Geometry check sheet. Reference: the model listing, model coordinates, mm. Face numbers are marked on the shaded views. A direction names the side the tool comes from. Give positions to 0.01 mm unless a question says otherwise; leave off trailing zeros. Order: outer loops, then holes, each group sorted by start corner. A loop starts at its lowest first (then second) coordinate and runs counter-clockwise, first axis right, second up. Notation, with made-up numbers: M 3.5,53 L 56.5,53 A22 cw 56.5,81 Z; hole C 60,33.25 d1. An arc over 180 degrees is marked long. Answer as CSV lines item,"result". Start each with the question number.
Q1. Section check B-B, the plane x = -50. Record the boundary of the cut face in (y, z).
Q2. Section check C-C, the plane x = -86. Record the boundary of the cut face in (y, z).
Q3. Go/stop test with flat-tipped pins: pin 1 (6 mm diameter, centred on x = -65, y = 16.5, fed in from +Z); pin 2 (5 mm diameter, centred on x = -80, y = 9.95, fed in from -Z); pin 3 (1.4 mm diameter, centred on y = 21.5, z = 1, fed in from +X); pin 4 (1.5 mm diameter, centred on x = -33.5, z = 1.5, fed in from -Y). Record where each tip stops, or that it passes through.
Q4. Section check A-A, the plane y = 16. Record the boundary of the cut face in (x, z).
Q5. Thickness scan on line 1 (Y direction, x = -70, z = 0.85); line 2 (Z direction, x = -87, y = 2.5); line 3 (X direction, y = 1.75, z = 0.95). Record the ranges inside material, lowest first.
Q6. Set-up check for the marked faces 1 and 2: record each of +Z, -Z, +X, -X, +Y, -Y from which the full face is reachable in a straight line by a thin tool's end or side.
```python
from build123d import *

# Parameters (mm, degrees)
F0_W      = 96
F0_H      = 20
F1_DEPTH  = 2.4
F4_DEPTH  = 20
F5_R      = 0.75
F6_DEPTH  = 20.001
F7_R      = 1.5
F8_DEPTH  = 2.401
F10_DEPTH = 2.4
F11_DEPTH = 2.401


with BuildPart() as f1:
    # F0 (on Top) → F1 (new body)
    with BuildSketch(Plane.XY):
        with Locations((-48, 10)):
            Rectangle(F0_W, F0_H)
    extrude(amount=F1_DEPTH)

    # F3 (on face) → F4 (join)
    with BuildSketch(Plane.XZ):
        with BuildLine():
            Line((-4.53507, 2.4), (0, 2.4))
            Line((0, 2.4), (0, 4.9))
            Line((0, 4.9), (-2.557698, 4.9))
            ThreePointArc((-2.557698, 4.9), (-3.861539, 4.416575), (-4.53507, 3.2))
            ThreePointArc((-4.53507, 3.2), (-4.769385, 2.634315), (-5.33507, 2.4))
            Line((-5.33507, 2.4), (-4.53507, 2.4))
        make_face()
    extrude(amount=-F4_DEPTH)

    # F5 (on face) → F6 (cut, through all)
    with BuildSketch(Plane.XZ):
        with Locations((-2.673816, 2.433896)):
            Circle(F5_R)
    extrude(amount=-F6_DEPTH, mode=Mode.SUBTRACT)

    # F7 (on face) → F8 (cut, through all)
    with BuildSketch(Plane.XY.offset(2.4)):
        with BuildLine():
            ThreePointArc((-91.5, 9.954306), (-90, 8.454306), (-88.5, 9.954306))
            ThreePointArc((-88.5, 9.954306), (-90, 11.454306), (-91.5, 9.954306))
        make_face()
        with Locations((-80, 9.954306)):
            Circle(F7_R)
        with Locations((-70, 9.954306)):
            Circle(F7_R)
        with Locations((-60, 9.954306)):
            Circle(F7_R)
        with Locations((-50, 9.954306)):
            Circle(F7_R)
        with Locations((-40, 9.954306)):
            Circle(F7_R)
    extrude(amount=-F8_DEPTH, mode=Mode.SUBTRACT)

    # F9 (on face) → F10 (join)
    with BuildSketch(Plane.XY.offset(2.4)):
        with BuildLine():
            Line((-95.2, 0), (-6, 0))
            Line((-6, 0), (-6, 20))
            Line((-6, 20), (-95.2, 20))
            ThreePointArc((-95.2, 20), (-95.765685, 20.234315), (-96, 20.8))
            Line((-96, 20.8), (-96, 22.5))
            ThreePointArc((-96, 22.5), (-96.234315, 23.065685), (-96.8, 23.3))
            Line((-96.8, 23.3), (-105.2, 23.3))
            ThreePointArc((-105.2, 23.3), (-105.765685, 23.065685), (-106, 22.5))
            Line((-106, 22.5), (-106, -2.5))
            ThreePointArc((-106, -2.5), (-105.765685, -3.065685), (-105.2, -3.3))
            Line((-105.2, -3.3), (-103.3, -3.3))
            Line((-103.3, -3.3), (-98.7, -3.3))
            Line((-98.7, -3.3), (-96.8, -3.3))
            ThreePointArc((-96.8, -3.3), (-96.234315, -3.065685), (-96, -2.5))
            Line((-96, -2.5), (-96, -0.8))
            ThreePointArc((-96, -0.8), (-95.765685, -0.234315), (-95.2, 0))
        make_face()
        with BuildLine():
            ThreePointArc((-103.550001, 19.2), (-103.315687, 19.765685), (-102.750001, 20))
            Line((-102.750001, 20), (-99.249999, 20))
            ThreePointArc((-99.249999, 20), (-98.684314, 19.765686), (-98.449999, 19.2))
            Line((-98.449999, 19.2), (-98.449999, 0.8))
            ThreePointArc((-98.449999, 0.8), (-98.684314, 0.234315), (-99.249999, 0))
            Line((-99.249999, 0), (-102.749999, 0))
            ThreePointArc((-102.749999, 0), (-103.315684, 0.234315), (-103.549999, 0.8))
            Line((-103.549999, 0.8), (-103.550001, 19.2))
        make_face(mode=Mode.SUBTRACT)
    extrude(amount=-F10_DEPTH)

    # F7 (on face) → F11 (cut, through all)
    with BuildSketch(Plane.XY.offset(2.4)):
        with BuildLine():
            ThreePointArc((-91.5, 9.954306), (-90, 8.454306), (-88.5, 9.954306))
            ThreePointArc((-88.5, 9.954306), (-90, 11.454306), (-91.5, 9.954306))
        make_face()
        with Locations((-80, 9.954306)):
            Circle(F7_R)
        with Locations((-70, 9.954306)):
            Circle(F7_R)
        with Locations((-60, 9.954306)):
            Circle(F7_R)
        with Locations((-50, 9.954306)):
            Circle(F7_R)
        with Locations((-40, 9.954306)):
            Circle(F7_R)
    extrude(amount=-F11_DEPTH, mode=Mode.SUBTRACT)


solid = f1.part
```
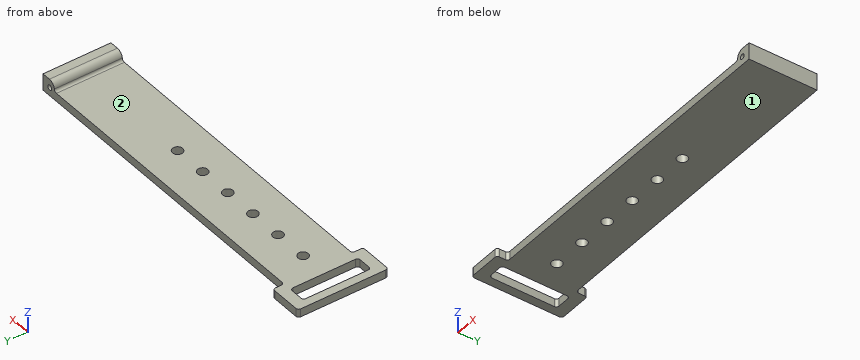
Answer block:
1,outline,"M 0,0 L 8.45,0 L 8.45,2.4 L 0,2.4 Z; M 11.45,0 L 20,0 L 20,2.4 L 11.45,2.4 Z"
2,outline,"M 0,0 L 20,0 L 20,2.4 L 0,2.4 Z"
3,pin 1,"stops at z = 2.4"
3,pin 2,"stops at z = 0"
3,pin 3,"stops at x = -96"
3,pin 4,"stops at y = 0"
4,outline,"M -106,0 L -103.55,0 L -103.55,2.4 L -106,2.4 Z; M -98.45,0 L 0,0 L 0,4.9 L -2.56,4.9 A2 ccw -4.54,3.2 A0.8 cw -5.34,2.4 L -98.45,2.4 Z; hole C -2.67,2.43 d1.5"
5,line 1,"y = 0 to 8.45, 11.45 to 20"
5,line 2,"z = 0 to 2.4"
5,line 3,"x = -106 to -103.55, -98.45 to 0"
6,face 1,"-Z, +X, -X, +Y, -Y"
6,face 2,"+Z, -X, +Y, -Y"
